Autodesk Inventor part; units mm, degrees
ref_plane "YZ Plane" through (0, 0, 0) normal (1, 0, 0) x (0, 1, 0)
ref_plane "XZ Plane" through (0, 0, 0) normal (0, 1, 0) x (-1, 0, 0)
ref_plane "XY Plane" through (0, 0, 0) normal (0, 0, 1) x (1, 0, 0)
sketch "Sketch3" plane through (0, 0, 0) normal (0, 0, 1) x (1, 0, 0)
  line L0 (-15.8918, -16.7) -> (15.8918, -16.7)
  line L1 (16.7, -15.7) -> (16.7, 15.7)
  line L2 (15.8918, 16.7) -> (-15.8918, 16.7)
  line L3 (-16.7, 15.7) -> (-16.7, -15.7)
  line L4 (-15.8918, 16.7) -> (-16.7, 15.7)
  line L5 (15.8918, 16.7) -> (16.7, 15.7)
  line L6 (16.7, -15.7) -> (15.8918, -16.7)
  line L7 (-16.7, -15.7) -> (-15.8918, -16.7)
  line L8 (-4.9497, -8.8994) -> (4.9497, -8.8994)
  line L9 (4.9497, -8.8994) -> (4.9497, 8.8994)
  line L10 (4.9497, 8.8994) -> (-4.9497, 8.8994)
  line L11 (-4.9497, 8.8994) -> (-4.9497, -8.8994)
  circle A0 centre (-12.14, 12.625) radius 2.045
  circle A1 centre (12.14, 12.625) radius 2.045
  line L12 (0, -16.7) -> (0, 16.7) construction
  circle A2 centre (-12.14, -12.625) radius 2.045
  circle A3 centre (12.14, -12.625) radius 2.045
  line L13 (12.14, 12.625) -> (-12.14, 12.625) construction
  line L14 (-12.14, 12.625) -> (-12.14, -12.625) construction
  line L15 (-12.14, -12.625) -> (12.14, -12.625) construction
  line L16 (12.14, -12.625) -> (12.14, 12.625) construction
  line L17 (-16.7, 0) -> (16.7, 0) construction
  circle A4 centre (0, 0) radius 18.4 construction
  circle A5 centre (-9, 4) radius 1.5
  circle A6 centre (9, 4) radius 1.5
  circle A7 centre (-9, -4) radius 1.5
  circle A8 centre (9, -4) radius 1.5
  dimension "d10" = 9.8994
  dimension "d11" = 17.7988
  dimension "d12" = 4.09
  dimension "d13" = 4.09
  dimension "d17" = 4.09
  dimension "d19" = 24.28
  dimension "d20" = 25.25
  dimension "d21" = 4.09
  dimension "d22" = 12.625
  dimension "d26" = 36.8
  dimension "d38" = 12.14
  dimension "d39" = 33.4
  dimension "d40" = 33.4
  dimension "d45" = 3
  dimension "d46" = 3
  dimension "d47" = 3
  dimension "d48" = 3
  dimension "d49" = 4
  dimension "d57" = 8.8994
  dimension "d58" = 4.9497
  dimension "d59" = 9
  dimension "d60" = 9
  dimension "d61" = 9
  dimension "d62" = 9
  dimension "d63" = 4
  dimension "d64" = 4
  dimension "d65" = 4
sketch "Sketch4" plane through (0, 0, 0) normal (0, 0, 1) x (1, 0, 0)
  circle A0 centre (0, 0) radius 12.7
  dimension "d32" = 25.4
extrude "Extrusion5" add sketch "Sketch3" along normal blind 8
extrude "Extrusion6" cut sketch "Sketch4" along normal blind 8 keep common part
properties part number "WG18FLANGECutDown" material "Brass, Soft Yellow"
Work out the finished part from the listing and answer in its coordinate system (mm). A direction names the side the tool comes from. Give positions to 0.01 mm unless a question says otherwise; leave off trailing zeros. Loops run counter-clockwise (first coordinate to the right, second up) from the corner with the lowest first, then second, coordinate; pieces in that order, holes last. Notation, with made-up numbers: (89, 54) - (128, 54) arc R8 cw to (128, 63) - close; hole circle Ø8 at (77, 24). An arc over 180 degrees is marked (long way). Use CSV: the item, a comma, the result in double quotes. Start each with the question number.
(1) Find section B-B, the plane y = 0. Determine the outline of the cut face in (x, z).
(2) Find section D-D, the plane x = 8. Determine the outline of the cut face in (y, z), plus the area to 3 significant figures.
(3) Each of these flat-tipped pins is pushed along its axis until it touches: pin 1 (1.5 mm diameter, centred on x = -2, y = 6.5, fed in from +Z); pin 2 (1.5 mm diameter, centred on x = -9.5, z = 4.5, fed in from -Y); pin 3 (2 mm diameter, centred on x = 2, z = 1.5, fed in from -Y). Where does it stop, or does it pass through?
(4) Find section C-C, the plane z = 1.25. Determine the outline of the cut face in (x, y), plus the area to 3 significant figures.
(5) Determine the mould class of faces 3 (the face through (5.5, 0.2, 8)), 4 (the face through (0, -8.899, 4)), 5 (the face through (-2.75, 12.4, 3.94)) for opening direction X: released by +X, released by -X, zero draft, split by the parting line, or undercut.
(6) Find section A-A, the plane x = 0. Determine the outline of the cut face in (y, z).
(7) Find the intervals of material crossed by L1, parallel to Y at x = 9.25, z = 7.25; L2, parallel to X at y = 3.75, z = 5.5; L3, parallel to Y at x = -9, z = 3.75, in increasing order.
(8) A tool of negligible diameter and unlimited length cuts with its end or side. For faces 1 (the face through (5.5, 0.2, 0)), 2 (the face through (4.95, 0, 4)), from which of +Z, -Z, +X, -X, +Y, -Y can it reach the whole face along a straight path? Write none if from no direction.
Results found:
1,outline,"(-12.7, 0) - (-4.95, 0) - (-4.95, 8) - (-12.7, 8) - close; (4.95, 0) - (12.7, 0) - (12.7, 8) - (4.95, 8) - close"
2,outline,"(-9.86, 0) - (-5.12, 0) - (-5.12, 8) - (-9.86, 8) - close; (-2.88, 0) - (2.88, 0) - (2.88, 8) - (-2.88, 8) - close; (5.12, 0) - (9.86, 0) - (9.86, 8) - (5.12, 8) - close"
2,area,"122 mm^2"
3,pin 1,"through"
3,pin 2,"y = -9.2"
3,pin 3,"y = -12.66"
4,outline,"circle Ø25.4 at (0, 0); hole circle Ø3 at (-9, -4); hole circle Ø3 at (-9, 4); hole (-4.95, -8.9) - (4.95, -8.9) - (4.95, 8.9) - (-4.95, 8.9) - close; hole circle Ø3 at (9, -4); hole circle Ø3 at (9, 4)"
4,area,"302 mm^2"
5,face 3,"zero draft"
5,face 4,"undercut"
5,face 5,"split by the parting line"
6,outline,"(-12.7, 0) - (-8.9, 0) - (-8.9, 8) - (-12.7, 8) - close; (8.9, 0) - (12.7, 0) - (12.7, 8) - (8.9, 8) - close"
7,L1,"-8.7 to -5.48, -2.52 to 2.52, 5.48 to 8.7"
7,L2,"-12.13 to -10.48, -7.52 to -4.95, 4.95 to 7.52, 10.48 to 12.13"
7,L3,"-8.96 to -5.5, -2.5 to 2.5, 5.5 to 8.96"
8,face 1,"-Z, +X, -X, +Y, -Y"
8,face 2,"+Z, -Z"
